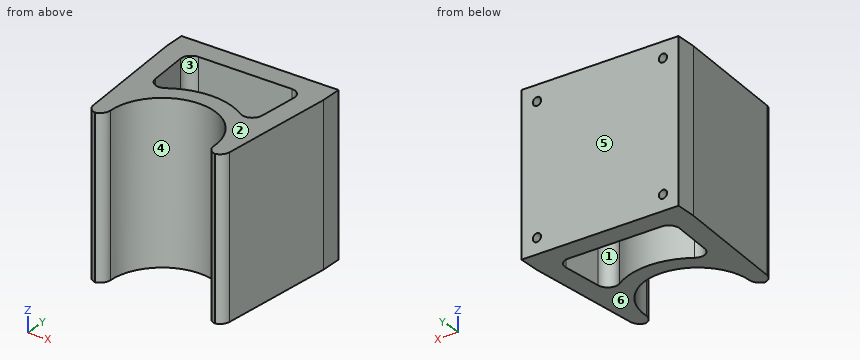
from build123d import *

# Parameters (mm, degrees)
SKETCH1_W                = 38
SKETCH1_H                = 38
BOSS_EXTRUDE1_DEPTH      = 5
F_2_0_2_DIAMETER_HOLE1_D = 2
BOSS_EXTRUDE3_START      = -19
BOSS_EXTRUDE3_DEPTH      = 38
BOSS_EXTRUDE4_START      = 19
BOSS_EXTRUDE4_DEPTH      = 38
FILLET5_START            = -20
FILLET5_DEPTH            = 40
FILLET5_START_2          = -19
FILLET5_2_DEPTH          = 38


with BuildPart() as part:
    # Sketch1 → Boss-Extrude1 (new body)
    with BuildSketch(Plane(origin=(0, 0, 0), x_dir=(1, 0, 0), z_dir=(0, 1, 0))):
        Rectangle(SKETCH1_W, SKETCH1_H)
    extrude(amount=BOSS_EXTRUDE1_DEPTH)

    # Ø2.0 (2) Diameter Hole1 (through all)
    with Locations(Plane(origin=(0, 5, 0), x_dir=(1, 0, 0), z_dir=(0, 1, 0))):
        with Locations((-15.25, 15.25), (15.25, 15.25), (15.25, -15.25), (-15.25, -15.25)):
            Hole(F_2_0_2_DIAMETER_HOLE1_D / 2)



with BuildPart() as body_2:
    # Sketch10 → Boss-Extrude3 (new body)
    with BuildSketch(Plane.XY.offset(BOSS_EXTRUDE3_START)):
        with BuildLine():
            Line((-12.247448714, -30.5), (-16.30950643, -30.5))
            ThreePointArc((-16.30950643, -30.5), (0, -11.5), (16.30950643, -30.5))
            Line((16.30950643, -30.5), (12.247448714, -30.5))
            ThreePointArc((12.247448714, -30.5), (0, -15.5), (-12.247448714, -30.5))
        make_face()
    extrude(amount=BOSS_EXTRUDE3_DEPTH)


with BuildPart() as part_1:
    add(part.part)

    add(body_2.part)  # Boss-Extrude4 merges body 2
    # Sketch11 → Boss-Extrude4 (add)
    with BuildSketch(Plane.XY.offset(BOSS_EXTRUDE4_START)):
        Polygon((-19, 0), (-16.30950643, -30.5), (-12.481964126, -17.208773398), (-14, 0), align=None)
    boss_extrude4 = extrude(amount=-BOSS_EXTRUDE4_DEPTH)

    # Mirror1: Boss-Extrude4 across plane
    add(boss_extrude4.mirror(Plane(origin=(0, 0, 0), x_dir=(0, 0, 1), z_dir=(1, 0, 0))))

    # Fillet5: read off the stored shape, not the designer's step
    # Fillet5 outline → Fillet5 (cut)
    with BuildSketch(Plane.XY.offset(FILLET5_START)):
        with BuildLine():
            ThreePointArc((16.51066015, -28.219679197), (15.881955848, -29.668637648), (14.510165322, -30.451542777))
            ThreePointArc((14.510165322, -30.451542777), (13.066791954, -29.585151934), (12.5, -28))
            ThreePointArc((12.5, -28), (12.436701913, -29.256362025), (12.247448714, -30.5))
            Line((12.247448714, -30.5), (16.30950643, -30.5))
            ThreePointArc((16.30950643, -30.5), (16.436174742, -29.449882703), (16.495299812, -28.393807221))
            Line((16.495299812, -28.393807221), (16.51066015, -28.219679197))
        make_face()
        with BuildLine():
            ThreePointArc((-12.247448714, -30.5), (-12.436701913, -29.256362025), (-12.5, -28))
            ThreePointArc((-12.5, -28), (-13.066791954, -29.585151934), (-14.510165322, -30.451542777))
            ThreePointArc((-14.510165322, -30.451542777), (-15.881955848, -29.668637648), (-16.51066015, -28.219679197))
            Line((-16.51066015, -28.219679197), (-16.495299812, -28.393807221))
            ThreePointArc((-16.495299812, -28.393807221), (-16.436174742, -29.449882703), (-16.30950643, -30.5))
            Line((-16.30950643, -30.5), (-12.247448714, -30.5))
        make_face()
    extrude(amount=FILLET5_DEPTH, mode=Mode.SUBTRACT)

    # Fillet5 2 outline → Fillet5 2 (add)
    with BuildSketch(Plane.XY.offset(FILLET5_START_2)):
        with BuildLine():
            Line((12.481964126, -17.208773398), (12.912072208, -12.33297787))
            ThreePointArc((12.912072208, -12.33297787), (11.511662087, -14.363204389), (9.050460767, -14.203654111))
            ThreePointArc((9.050460767, -14.203654111), (10.870557296, -15.587063841), (12.481964126, -17.208773398))
        make_face()
        with BuildLine():
            ThreePointArc((11.269759694, 0), (13.113559845, -0.811686936), (13.7600892, -2.719679197))
            Line((13.7600892, -2.719679197), (14, 0))
            Line((14, 0), (11.269759694, 0))
        make_face()
        with BuildLine():
            ThreePointArc((-12.481964126, -17.208773398), (-10.870557296, -15.587063841), (-9.050460767, -14.20365411))
            ThreePointArc((-9.050460767, -14.20365411), (-11.511662087, -14.363204389), (-12.912072208, -12.33297787))
            Line((-12.912072208, -12.33297787), (-12.481964126, -17.208773398))
        make_face()
        with BuildLine():
            ThreePointArc((-13.7600892, -2.719679197), (-13.113559845, -0.811686936), (-11.269759694, 0))
            Line((-11.269759694, 0), (-14, 0))
            Line((-14, 0), (-13.7600892, -2.719679197))
        make_face()
    extrude(amount=FILLET5_2_DEPTH)


solid = part_1.part
Check sheet for the modelled part. Datum: model origin and axes. Units: mm. Face numbers are marked on the shaded views. A direction names the side the tool comes from. Round coordinates to 2 decimals unless told otherwise and drop trailing zeros. Loops run counter-clockwise (first coordinate to the right, second up) from the corner with the lowest first, then second, coordinate; pieces in that order, holes last. Notation, with made-up numbers: (74, -22.75) -> (79, -22.75) arc R32 ccw to (79, 11.25) -> close; hole circle Ø9 at (59.5, 7). An arc over 180 degrees is marked (long way). Put each result on its own line as item: value. Start each with the question number.
1. Section check C-C (y = -9.5). Enter the section's corners in (x, z), plus the area to 3 significant figures.
2. Access from +Z, -Z, +X, -X, +Y, -Y to the whole of each face (thin tool, end or side, straight path). Record for the marked faces 1 and 2.
3. Scan lines: probe 1 along X at (y, z) = (1.95, -15.25); probe 2 along X at (y, z) = (-3, -13.5). Record each from-to range of solid material in increasing order.
4. Draft check along Y on the marked faces 3, 4, 5 and 6. Enter one of: +Y half, -Y half, draft (parallel to the pull), parting line (faces both ways), or undercut.
5. Section check D-D (z = -8). Enter the section's corners in (x, y).
6. Section check B-B (z = -15.25). Enter the section's corners in (x, y).
7. Section check A-A (x = 0). Enter the section's corners in (y, z), plus the area to 3 significant figures.
8. Gauge pin test, flat ends, axial feed: pin 1 (10 mm diameter, centred on x = 13, z = -3.5, fed in from -Y); pin 2 (0.6 mm diameter, centred on x = 15.5, z = -15.5, fed in from +Y). Record the tip position at first contact, or that the pin passes through.
Findings:
1. outline: (-18.16, -19) -> (-13.16, -19) -> (-13.16, 19) -> (-18.16, 19) -> close; (13.16, -19) -> (18.16, -19) -> (18.16, 19) -> (13.16, 19) -> close
1. area: 380 mm^2
2. face 1: +Z, -Z
2. face 2: +Z, +X, -X, +Y, -Y
3. probe 1: x = -19 to -16.25, -14.25 to 14.25, 16.25 to 19
3. probe 2: x = -18.74 to -13.74, 13.74 to 18.74
4. face 3: undercut
4. face 4: -Y half
4. face 5: +Y half
4. face 6: draft
5. outline: (-19, 0) -> (-16.51, -28.22) arc R2.5 ccw to (-14.51, -30.45) arc R2.5 ccw to (-12.5, -28) arc R12.5 cw to (12.5, -28) arc R2.5 ccw to (14.51, -30.45) arc R2.5 ccw to (16.51, -28.22) -> (19, 0) -> (19, 5) -> (-19, 5) -> close; hole (-13.76, -2.72) -> (-12.91, -12.33) arc R2.5 ccw to (-9.05, -14.2) arc R16.5 cw to (9.05, -14.2) arc R2.5 ccw to (12.91, -12.33) -> (13.76, -2.72) arc R2.5 ccw to (11.27, 0) -> (-11.27, 0) arc R2.5 ccw to start
6. outline: (-19, 0) -> (-16.51, -28.22) arc R2.5 ccw to (-14.51, -30.45) arc R2.5 ccw to (-12.5, -28) arc R12.5 cw to (12.5, -28) arc R2.5 ccw to (14.51, -30.45) arc R2.5 ccw to (16.51, -28.22) -> (19, 0) -> (19, 5) -> (16.25, 5) -> (16.25, 0) -> (14.25, 0) -> (14.25, 5) -> (-14.25, 5) -> (-14.25, 0) -> (-16.25, 0) -> (-16.25, 5) -> (-19, 5) -> close; hole (-13.76, -2.72) -> (-12.91, -12.33) arc R2.5 ccw to (-9.05, -14.2) arc R16.5 cw to (9.05, -14.2) arc R2.5 ccw to (12.91, -12.33) -> (13.76, -2.72) arc R2.5 ccw to (11.27, 0) -> (-11.27, 0) arc R2.5 ccw to start
7. outline: (-15.5, -19) -> (-11.5, -19) -> (-11.5, 19) -> (-15.5, 19) -> close; (0, -19) -> (5, -19) -> (5, 19) -> (0, 19) -> close
7. area: 342 mm^2
8. pin 1: stops at y = -30.45
8. pin 2: stops at y = 0
